Geometry check sheet. Reference: the model listing, model coordinates, mm. Face numbers are marked on the shaded views. A direction names the side the tool comes from. Round coordinates to 2 decimals unless told otherwise and drop trailing zeros. Loops run counter-clockwise (first coordinate to the right, second up) from the corner with the lowest first, then second, coordinate; pieces in that order, holes last. Notation, with made-up numbers: M 84.25,30.5 L 135.25,30.5 A14 cw 135.25,42.5 Z; hole C 14,-39 d4. An arc over 180 degrees is marked long. Use one line per item in the form item = value. Start each with the question number.
1. Cross-section at B-B (x = -7). Record the boundary of the cut face in (y, z).
2. Set-up check for the marked faces 1, 2 and 3: record each of +Z, -Z, +X, -X, +Y, -Y from which the full face is reachable in a straight line by a thin tool's end or side.
3. Cross-section at C-C (x = 0). Record the boundary of the cut face in (y, z).
4. Go/stop test with flat-tipped pins: pin 1 (3 mm diameter, centred on x = 9.5, z = 2, fed in from -Y); pin 2 (3 mm diameter, centred on x = 26, y = -14, fed in from +Z); pin 3 (3 mm diameter, centred on x = 21.5, y = -10, fed in from +Z). Record where each tip stops, or that it passes through.
5. Cross-section at A-A (z = -1). Record the boundary of the cut face in (x, y).
6. Cross-section at D-D (y = -1.25). Record the boundary of the cut face in (x, z).
7. Material ranges on line 1 (Z direction, x = -3, y = -2); line 2 (Y direction, x = -7, z = -4.15); line 3 (X direction, y = -8.25, z = 0.25), recorded low to high.
8. Draft check along Y on the marked faces 4, 5, 6 and 7. Enter one of: pulls with the +Y half, pulls with the -Y half, needs draft (parallel to the pull), parting line crosses it, or undercut.
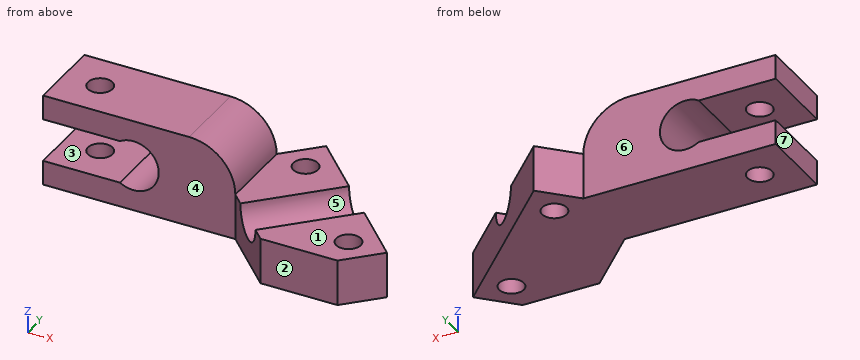
```python
from build123d import *

# Parameters (mm, degrees)
PAD_DEPTH            = 10
SKETCH_R             = 1.6
PAD001_DEPTH         = 6
SKETCH004_R          = 3
POCKET_DEPTH         = 27.372693
SKETCH005_R          = 1.6
POCKET001_DEPTH      = 6.001
POCKET001_DEPTH_BACK = -6.001


with BuildPart() as part:
    # Sketch003 → Pad (new body)
    with BuildSketch(Plane.XZ):
        with BuildLine():
            Line((13.253575, -6), (-11.746425, -6))
            Line((-11.746425, -2.8), (-11.746425, -6))
            Line((-1.746425, -2.8), (-11.746425, -2.8))
            ThreePointArc((-1.746425, -2.8), (3.3, 0), (-1.746425, 2.8))
            Line((-1.746425, 2.8), (-11.746425, 2.8))
            Line((-11.746425, 2.8), (-11.746425, 6))
            Line((7.253575, 6), (-11.746425, 6))
            ThreePointArc((13.253575, 0), (11.496216, 4.242641), (7.253575, 6))
            Line((13.253575, 0), (13.253575, -6))
        make_face()
    extrude(amount=PAD_DEPTH)

    # Sketch → Pad001 (join)
    with BuildSketch(Plane.XY):
        Polygon((13.253575, -10), (20.324643, -17.071068), (30.324643, -17.071068), (34.517031, -12.87868), (17.445963, 4.192388), (13.253575, 0), align=None)
        with Locations((17.445963, -0.807612)):
            Circle(SKETCH_R, mode=Mode.SUBTRACT)
        with Locations((29.517031, -12.87868)):
            Circle(SKETCH_R, mode=Mode.SUBTRACT)
    extrude(amount=-PAD001_DEPTH)

    # Sketch004 (on DatumPlane) → Pocket (cut, through all)
    with BuildSketch(Plane(origin=(0, 0, 3.5), x_dir=(0, 0, -1), z_dir=(-0.707107, -0.707107, 0))):
        with Locations((3.5, 21.442761)):
            Circle(SKETCH004_R)
    extrude(amount=-POCKET_DEPTH, mode=Mode.SUBTRACT)

    # Sketch005 → Pocket001 (cut, two sides)
    with BuildSketch(Plane.XY) as pocket001_sk:
        with Locations((-7, -5)):
            Circle(SKETCH005_R)
    extrude(amount=-POCKET001_DEPTH, mode=Mode.SUBTRACT)
    extrude(pocket001_sk.sketch, amount=-POCKET001_DEPTH_BACK, mode=Mode.SUBTRACT)


solid = part.part
```
Reported:
q1.outline = M -10,-6 L -6.6,-6 L -6.6,-2.8 L -10,-2.8 Z; M -10,2.8 L -6.6,2.8 L -6.6,6 L -10,6 Z; M -3.4,-6 L 0,-6 L 0,-2.8 L -3.4,-2.8 Z; M -3.4,2.8 L 0,2.8 L 0,6 L -3.4,6 Z
q2.face_1 = +Z, +X, +Y, -Y
q2.face_2 = +Z, -Z, +X, -X, -Y
q2.face_3 = -X, +Y, -Y
q3.outline = M -10,-6 L 0,-6 L 0,-3.3 L -10,-3.3 Z; M -10,3.3 L 0,3.3 L 0,6 L -10,6 Z
q4.pin_1 = -10
q4.pin_2 = 0
q4.pin_3 = -1.89
q5.outline = M 3.14,-10 L 13.25,-10 L 14.79,-11.54 L 23.98,-2.34 L 17.45,4.19 L 13.25,0 L 3.14,0 Z; M 18.79,-15.54 L 20.32,-17.07 L 30.32,-17.07 L 34.52,-12.88 L 27.98,-6.34 Z; hole C 17.45,-0.81 d3.2; hole C 29.52,-12.88 d3.2
q6.outline = M -11.75,-6 L 15.91,-6 L 15.91,0 L 13.25,0 A6 ccw 7.25,6 L -11.75,6 L -11.75,2.8 L -1.75,2.8 A3.3 cw long -1.75,-2.8 L -11.75,-2.8 Z; M 18.98,-6 L 22.89,-6 L 22.89,0 L 18.98,0 Z
q7.line_1 = -6 to -2.8, 2.8 to 6
q7.line_2 = -10 to -6.6, -3.4 to 0
q7.line_3 = 3.29 to 13.25
q8.face_4 = pulls with the -Y half
q8.face_5 = undercut
q8.face_6 = pulls with the +Y half
q8.face_7 = needs draft
